Check sheet for the modelled part. Datum: model origin and axes. Units: mm. A direction names the side the tool comes from. Round coordinates to 2 decimals unless told otherwise and drop trailing zeros. Order: outer loops, then holes, each group sorted by start corner. A loop starts at its lowest first (then second) coordinate and runs counter-clockwise, first axis right, second up.
(1) Mould release check, pull along X, two halves, no side actions. Record for faces 4 (the flat face through (2.39, 1.18, -1.36)), 5 (the cylindrical face through (0.45, 1.97, 1.43)), 6 (the flat face through (1.45, 2.4, 2.52)): released by +X, released by -X, zero draft, split by the parting line, or undercut.
(2) Thickness scan on probe 1 along X at (y, z) = (2.8, 0); probe 2 along X at (y, z) = (2.25, 0.7); probe 3 along Y at (x, z) = (2.75, -0.5). Record the ranges inside material, lowest first.
(3) Tool access check on faces 1 (the flat face through (1.45, 2.4, -2.52)), 2 (the flat face through (-1.5, 2.4, 2.5)), 3 (the cylindrical face through (-2.685, 2.942, -0.596)). Record the directions out of +Z, -Z, +X, -X, +Y, -Y that give a thin tool (end or side, any length) a straight path to the whole face; none if there is none.
(4) Sectioned sample at A-A, the plane y = 1.75. Enter the section's corners in (x, z).
(5) Sectioned sample at B-B, the plane y = 2.55. Enter the section's corners in (x, z), and give its area (3 significant figures).
```python
from build123d import *

# Parameters (mm, degrees)
ESQUISSE1_R        = 1.5
BOSS_EXTRU_1_DEPTH = 2.4
ESQUISSE2_R        = 2.75
ESQUISSE2_R_2      = 1.5
BOSS_EXTRU_2_DEPTH = 1.6
CONG_1_R           = 0.5


with BuildPart() as part:
    # Esquisse1 → Boss.-Extru.1 (new body)
    with BuildSketch(Plane(origin=(0, 0, 0), x_dir=(1, 0, 0), z_dir=(0, 1, 0))):
        Polygon((3.175426481, 0), (1.58771324, 2.75), (-1.58771324, 2.75), (-3.175426481, 0), (-1.58771324, -2.75), (1.58771324, -2.75), align=None)
        with Locations(Location((0, 0, 0), (0, 0, 270))):
            Circle(ESQUISSE1_R, mode=Mode.SUBTRACT)
    extrude(amount=BOSS_EXTRU_1_DEPTH)

    # Esquisse2 → Boss.-Extru.2 (add)
    with BuildSketch(Plane(origin=(0, 2.4, 0), x_dir=(1, 0, 0), z_dir=(0, 1, 0))):
        with Locations(Location((0, 0, 0), (0, 0, 270))):
            Circle(ESQUISSE2_R)
        with Locations(Location((0, 0, 0), (0, 0, 270))):
            Circle(ESQUISSE2_R_2, mode=Mode.SUBTRACT)
    extrude(amount=BOSS_EXTRU_2_DEPTH)

    # Congé1
    cong_1_edges = [part.edges().sort_by_distance(p)[0] for p in [
        (0, 4, -2.75),
    ]]
    fillet(cong_1_edges, radius=CONG_1_R)


solid = part.part
```
Derived:
1. face 4: released by +X
1. face 5: undercut
1. face 6: zero draft
2. probe 1: x = -2.75 to -1.5, 1.5 to 2.75
2. probe 2: x = -2.77 to -1.33, 1.33 to 2.77
2. probe 3: y = 0 to 2.4
3. face 1: -Z, +X, +Y
3. face 2: +Z, -X, +Y
3. face 3: +Y
4. outline: (-3.18, 0) - (-1.59, -2.75) - (1.59, -2.75) - (3.18, 0) - (1.59, 2.75) - (-1.59, 2.75) - close; hole circle Ø3 at (0, 0)
5. outline: circle Ø5.5 at (0, 0); hole circle Ø3 at (0, 0)
5. area: 16.7 mm2
